Geometry check sheet. Reference: the model listing, model coordinates, mm. A direction names the side the tool comes from. Round coordinates to 2 decimals unless told otherwise and drop trailing zeros. Write each loop counter-clockwise with the first axis right and the second up, starting at its lowest first coordinate (ties: lowest second). Pieces come first, ordered by that corner, then holes. Notation, with made-up numbers: M 40.25,64.5 L 78.25,64.5 A28 ccw 78.25,102.5 Z; hole C 50,85.5 d10. An arc over 180 degrees is marked long. Use a Markdown table: item, result.
```python
from build123d import *

# Parameters (mm, degrees)
SKETCH020_W     = 74.5
SKETCH020_H     = 106.5
SKETCH020_W_2   = 56.5
SKETCH020_H_2   = 86.5
PAD009_DEPTH    = 5.2
SKETCH021_W     = 74.5
SKETCH021_H     = 106.5
PAD010_DEPTH    = 2
SKETCH022_R     = 1.45
POCKET011_DEPTH = 9


with BuildPart() as part:
    # Sketch020 (on ShapeBinder) → Pad009 (new body)
    with BuildSketch(Plane.YX.offset(-46)):
        with Locations((43.85, 111.75)):
            Rectangle(SKETCH020_W, SKETCH020_H)
        with Locations((43.85, 111.75)):
            Rectangle(SKETCH020_W_2, SKETCH020_H_2, mode=Mode.SUBTRACT)
    extrude(amount=PAD009_DEPTH)

    # Sketch021 (on Face10 of Pad009) → Pad010 (join)
    with BuildSketch(Plane.YX.offset(-40.8)):
        with Locations((43.85, 111.75)):
            Rectangle(SKETCH021_W, SKETCH021_H)
        Polygon((67.1, 149.6), (15.6, 149.6), (15.6, 112), (19.1, 112), (19.1, 88.5), (67.1, 88.5), align=None, mode=Mode.SUBTRACT)
    extrude(amount=PAD010_DEPTH)

    # Sketch022 (on Face4 of Pad010) → Pocket011 (cut)
    with BuildSketch(Plane(origin=(0, 0, 46), x_dir=(0, -1, 0), z_dir=(0, 0, 1))):
        with Locations((-76.6, 159.5)):
            Circle(SKETCH022_R)
        with Locations((-11.6, 159.5)):
            Circle(SKETCH022_R)
        with Locations((-11.6, 64.5)):
            Circle(SKETCH022_R)
        with Locations((-76.6, 64.5)):
            Circle(SKETCH022_R)
    extrude(amount=-POCKET011_DEPTH, mode=Mode.SUBTRACT)


solid = part.part
```
Item 1: Cross-section at A-A, the plane y = 36.5. Record the cut outline in (x, z), and give its area (3 significant figures).
Outcome:
| item | result |
|---|---|
| outline | M 58.5,38.8 L 88.5,38.8 L 88.5,40.8 L 68.5,40.8 L 68.5,46 L 58.5,46 Z; M 149.6,38.8 L 165,38.8 L 165,46 L 155,46 L 155,40.8 L 149.6,40.8 Z |
| area | 195 mm2 |
Item 2: Cross-section at D-D, the plane z = 43.75. Record the cut outline in (x, y).
Outcome:
| item | result |
|---|---|
| outline | M 58.5,6.6 L 165,6.6 L 165,81.1 L 58.5,81.1 Z; hole C 64.5,11.6 d2.9; hole C 64.5,76.6 d2.9; hole M 68.5,15.6 L 155,15.6 L 155,72.1 L 68.5,72.1 Z; hole C 159.5,11.6 d2.9; hole C 159.5,76.6 d2.9 |
Item 3: Material ranges on line 1 along X through (y, z) = (76.6, 41); line 2 along Y through (x, z) = (159.5, 41); line 3 along Y through (x, z) = (90.5, 45.75), recorded low to high. Write a range as from..to.
Outcome:
| item | result |
|---|---|
| line 1 | x = 58.5..63.05, 65.95..158.05, 160.95..165 |
| line 2 | y = 6.6..10.15, 13.05..75.15, 78.05..81.1 |
| line 3 | y = 6.6..15.6, 72.1..81.1 |
Item 4: Mould release check, pull along X, two halves, no side actions. Record for faces 1 (the face through (120, 13, 46)), 2 (the face through (112, 17, 40)), 3 (the face through (68.5, 43, 43)), 4 (the face through (58.5, 43, 42)): +X half, -X half, draft (parallel to the pull), parting line (faces both ways), or undercut.
Outcome:
| item | result |
|---|---|
| face 1 | draft |
| face 2 | undercut |
| face 3 | undercut |
| face 4 | -X half |
Item 5: Cross-section at B-B, the plane x = 138.5. Record the cut outline in (y, z), and give its area (3 significant figures).
Outcome:
| item | result |
|---|---|
| outline | M 6.6,38.8 L 15.6,38.8 L 15.6,46 L 6.6,46 Z; M 67.1,38.8 L 81.1,38.8 L 81.1,46 L 72.1,46 L 72.1,40.8 L 67.1,40.8 Z |
| area | 140 mm2 |
Item 6: Access from +Z, -Z, +X, -X, +Y, -Y to the whole of each face (thin tool, end or side, straight path). Record for faces 5 (the face through (101, 68, 38.8)), 6 (the face through (149.6, 42, 40)), 7 (the face through (111, 72.1, 43)).
Outcome:
| item | result |
|---|---|
| face 5 | -Z, +X, -X, +Y, -Y |
| face 6 | +Z, -Z |
| face 7 | +Z |
Item 7: Cross-section at C-C, the plane x = 64.5. Record the cut outline in (y, z), and give its area (3 significant figures).
Outcome:
| item | result |
|---|---|
| outline | M 6.6,38.8 L 10.15,38.8 L 10.15,46 L 6.6,46 Z; M 13.05,38.8 L 75.15,38.8 L 75.15,46 L 13.05,46 Z; M 78.05,38.8 L 81.1,38.8 L 81.1,46 L 78.05,46 Z |
| area | 495 mm2 |
